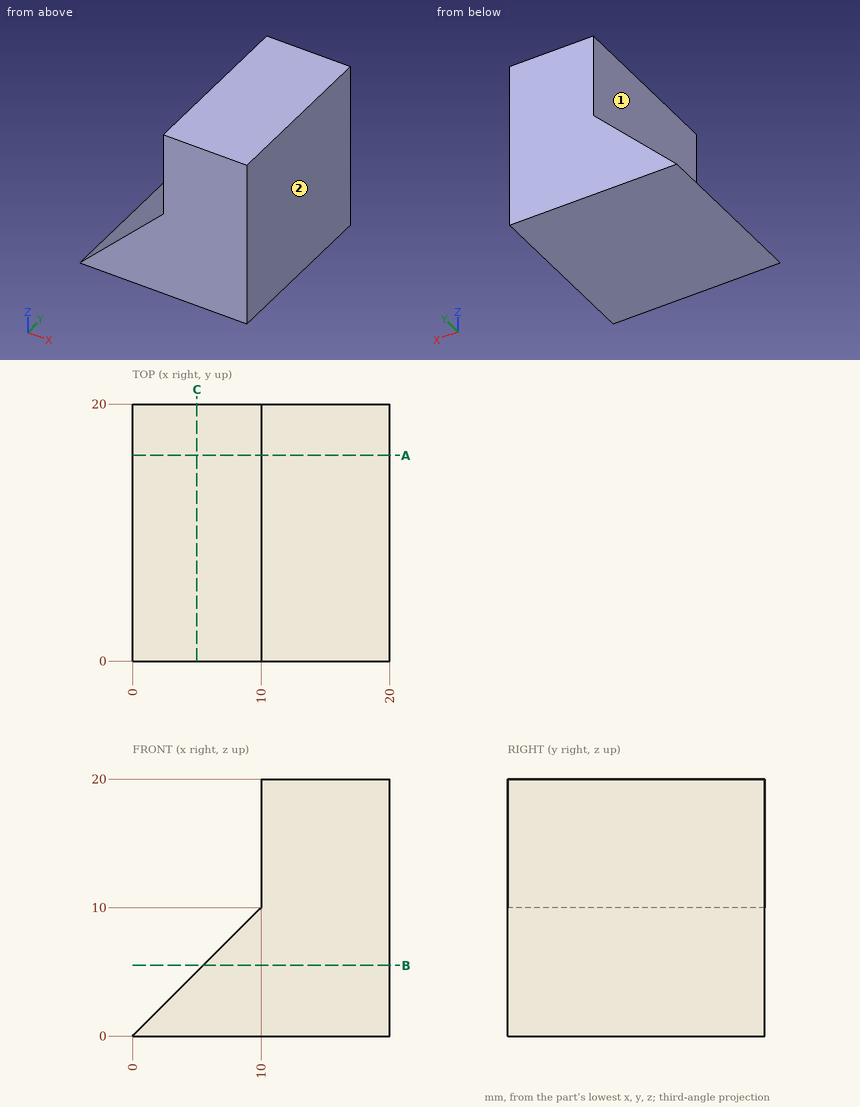
Study the drawing (mm; zero at the part's minimum x, y, z) and answer. A direction names the side the tool comes from. Round coordinates to 2 decimals unless told otherwise and drop trailing zeros. Write each loop counter-clockwise with the first axis right and the second up, starting at its lowest first coordinate (ties: lowest second). Pieces come first, ordered by that corner, then holes.
1) Given pin 1 Ø5 at (y, z) = (10.5, 14) entering from -X; pin 2 Ø1 at (x, y) = (5.5, 5.5) entering from +Z, each flat-ended and moving along its own axis, determine where each tip first touches the part or whether it passes through.
2) A cutting plane is placed at B-B (z = 5.5). Give the vertices of the cut face in (x, y), plus the area to 3 significant figures.
3) A tool of negligible diameter and unlimited length cuts with its end or side. For the marked faces 1 and 2, from which of +Z, -Z, +X, -X, +Y, -Y can it reach the whole face along a straight path? Write none if from no direction.
4) A cutting plane is placed at A-A (y = 16). Give the vertices of the cut face in (x, z).
5) A cutting plane is placed at C-C (x = 5). Give the vertices of the cut face in (y, z), plus the area to 3 significant figures.
6) Straight lines are drawn through the part: line 1 (X direction, y = 6.5, z = 12); line 2 (X direction, y = 15, z = 8); line 3 (Z direction, x = 4, y = 7.5). For each, find the intervals that lie inside material, in ascending order.
Completed:
1. pin 1: stops at x = 10
1. pin 2: stops at z = 6
2. outline: (5.5, 0) - (20, 0) - (20, 20) - (5.5, 20) - close
2. area: 290 mm2
3. face 1: +Z, -X, +Y, -Y
3. face 2: +Z, -Z, +X, +Y, -Y
4. outline: (0, 0) - (20, 0) - (20, 20) - (10, 20) - (10, 10) - close
5. outline: (0, 0) - (20, 0) - (20, 5) - (0, 5) - close
5. area: 100 mm2
6. line 1: x = 10 to 20
6. line 2: x = 8 to 20
6. line 3: z = 0 to 4
